Could you check a few things on this model? Use its own coordinates, in mm. Face numbers are marked on the shaded views. A direction names the side the tool comes from. Round coordinates to 2 decimals unless told otherwise and drop trailing zeros. Write each loop counter-clockwise with the first axis right and the second up, starting at its lowest first coordinate (ties: lowest second). Pieces come first, ordered by that corner, then holes. Notation, with made-up numbers: (-29, 59.5) -> (-21, 59.5) arc R26 ccw to (-21, 84.5) -> close; hole circle Ø2 at (67, 29.5). An arc over 180 degrees is marked (long way). One line per question, with ' | ' between items. Start each with the question number.
1. Imagine slicing it at A-A, the plane y = -21.25. List the corners of the cut face in (x, z) for me, and give its area (3 significant figures).
2. For pin 1 Ø6.5 at (x, y) = (-11.5, -11.5) entering from +Z; pin 2 Ø1 at (y, z) = (-11.5, 18.5) entering from +X, each with a flat end and sliding along its axis, tell me the tip position at first contact or that it passes through.
3. Imagine slicing it at B-B, the plane x = -10. List the corners of the cut face in (y, z) for me.
4. If I drill on line 1 along Z through (x, y) = (-11, -8.25); line 2 along X through (y, z) = (-9.75, 20); line 3 along X through (y, z) = (-5, 18.75), over which ranges is the centre line in solid material (lowest first)? Write a range as [from, to].
5. Imagine slicing it at C-C, the plane z = 16.5. List the corners of the cut face in (x, y) for me.
6. For the marked faces 1 and 2, which set-ups out of +Z, -Z, +X, -X, +Y, -Y let a thin tool reach every point of the face, with its end or its side?
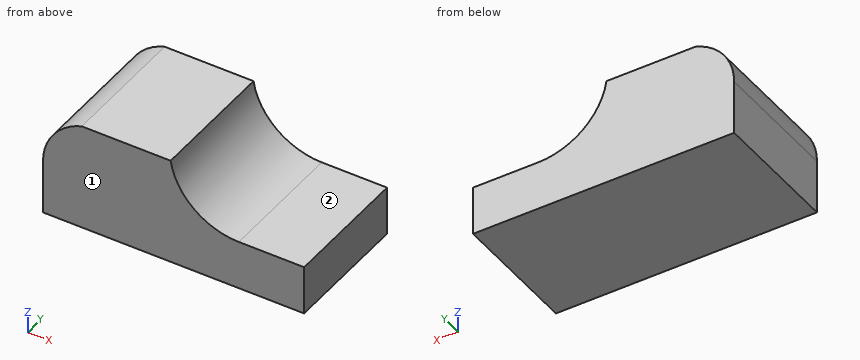
from build123d import *

# Parameters (mm, degrees)
F1_DEPTH = 25.4
F3_DEPTH = 25.4


with BuildPart() as f1:
    # F0 (on Front) → F1 (new body)
    with BuildSketch(Plane.XZ):
        with BuildLine():
            Line((-56.592982, 10.47193), (-56.592982, 0))
            Line((-56.592982, 0), (-5.792982, 0))
            Line((-5.792982, 0), (-5.792982, 9.580702))
            Line((-5.792982, 9.580702), (-18.492982, 9.580702))
            ThreePointArc((-18.492982, 9.580702), (-27.683477, 12.761842), (-32.940801, 20.943859))
            Line((-32.940801, 20.943859), (-50.7854, 20.943859))
            ThreePointArc((-50.7854, 20.943859), (-55.017084, 16.562817), (-56.592982, 10.679176))
            Line((-56.592982, 10.679176), (-56.592982, 10.47193))
        make_face()
        with BuildLine():
            ThreePointArc((-56.592982, 10.679176), (-56.593423, 10.575553), (-56.592982, 10.47193))
            Line((-56.592982, 10.47193), (-56.592982, 10.679176))
        make_face()
        with BuildLine():
            Line((-56.592982, 20.943859), (-56.592982, 10.679176))
            ThreePointArc((-56.592982, 10.679176), (-55.017084, 16.562817), (-50.7854, 20.943859))
            Line((-50.7854, 20.943859), (-56.592982, 20.943859))
        make_face()
        with BuildLine():
            ThreePointArc((-32.940801, 20.943859), (-27.683477, 12.761842), (-18.492982, 9.580702))
            Line((-18.492982, 9.580702), (-18.492982, 20.943859))
            Line((-18.492982, 20.943859), (-32.940801, 20.943859))
        make_face()
    extrude(amount=F1_DEPTH)

    # F2 (on face) → F3 (cut)
    with BuildSketch(Plane.XZ.offset(25.4)):
        with BuildLine():
            ThreePointArc((-56.592982, 10.679176), (-54.5049, 17.047845), (-49.051359, 20.943859))
            Line((-49.051359, 20.943859), (-56.592982, 20.943859))
            Line((-56.592982, 20.943859), (-56.592982, 10.679176))
        make_face()
        with BuildLine():
            Line((-18.492982, 20.943859), (-31.762764, 20.943859))
            ThreePointArc((-31.762764, 20.943859), (-27.22809, 12.809668), (-18.492982, 9.580702))
            Line((-18.492982, 9.580702), (-18.492982, 20.943859))
        make_face()
    extrude(amount=-F3_DEPTH, mode=Mode.SUBTRACT)


solid = f1.part
Geometry results:
1) outline: (-56.59, 0) -> (-5.79, 0) -> (-5.79, 9.58) -> (-18.49, 9.58) arc R13.43 cw to (-31.76, 20.94) -> (-49.05, 20.94) arc R10.76 ccw to (-56.59, 10.68) arc R12.17 ccw to (-56.59, 10.47) -> close | area: 785 mm2
2) pin 1: stops at z = 9.58 | pin 2: stops at x = -30.95
3) outline: (-25.4, 0) -> (0, 0) -> (0, 9.58) -> (-25.4, 9.58) -> close
4) line 1: z = [0, 9.58] | line 2: x = [-51.21, -31.58] | line 3: x = [-52.95, -31.23]
5) outline: (-54.88, -25.4) -> (-30.24, -25.4) -> (-30.24, 0) -> (-54.88, 0) -> close
6) face 1: +Z, -Z, +X, -X, -Y | face 2: +Z, +X, +Y, -Y
